from build123d import *

# Parameters (mm, degrees)
SKETCH_1_R      = 6
EXTRUDE_1_DEPTH = 3
SKETCH_2_R      = 3
EXTRUDE_2_DEPTH = 15.8
FILLET_1_R      = 1
FILLET_2_R      = 1.5


with BuildPart() as part:
    # ｽｹｯﾁ1 → ﾎﾞｽ - 押し出し1 (new body)
    with BuildSketch(Plane(origin=(0, 0, 0), x_dir=(1, 0, 0), z_dir=(0, 1, 0))):
        Circle(SKETCH_1_R)
    extrude(amount=EXTRUDE_1_DEPTH)

    # ｽｹｯﾁ2 → ﾎﾞｽ - 押し出し2 (add)
    with BuildSketch(Plane(origin=(0, 3, 0), x_dir=(1, 0, 0), z_dir=(0, 1, 0))):
        Circle(SKETCH_2_R)
    extrude(amount=EXTRUDE_2_DEPTH)

    # ﾌｨﾚｯﾄ1
    fillet_1_edges = [part.edges().sort_by_distance(p)[0] for p in [
        (-3, 18.8, 0),
    ]]
    fillet(fillet_1_edges, radius=FILLET_1_R)

    # ﾌｨﾚｯﾄ2
    fillet_2_edges = [part.edges().sort_by_distance(p)[0] for p in [
        (-6, 0, 0),
    ]]
    fillet(fillet_2_edges, radius=FILLET_2_R)


solid = part.part
For this review, take the finished solid that the model builds, in its own axes (mm). A direction names the side the tool comes from. Round coordinates to 2 decimals unless told otherwise and drop trailing zeros. Write each loop counter-clockwise with the first axis right and the second up, starting at its lowest first coordinate (ties: lowest second). Pieces come first, ordered by that corner, then holes. Notation, with made-up numbers: M 78,-22.75 L 85,-22.75 A25 cw 85,-5.75 Z; hole C 62,36 d11. An arc over 180 degrees is marked long. Write item = value, one per line. Start each with the question number.
(1) For faces 1 (the face through (-3, 3, 1)), 2 (the face through (0, 0, 0)), list the 3-axis set-ups (+Z, -Z, +X, -X, +Y, -Y) from which the entire face can be reached by the end or side of a thin tool; tool diameter is ignored.
(2) We need section A-A (x = 0). Give the boundary of the cut face in (y, z).
(3) We need section C-C (y = 15). Give the boundary of the cut face in (x, z), then the cut area to 3 significant figures.
(4) For line 1 along X through (y, z) = (6, 0); line 2 along Y through (x, z) = (3.5, -3); line 3 along Y through (x, z) = (0.75, -2.25), list the stretches that pass through material, from the lowest coordinate up.
(5) We need section B-B (z = 0). Give the boundary of the cut face in (x, y).
(6) Clearance check with flat-ended pins moving along their axes: pin 1 Ø1 at (x, z) = (1.5, -0.5) entering from -Y; pin 2 Ø4 at (x, y) = (4.5, 2.5) entering from -Z; pin 3 Ø3 at (y, z) = (3.5, -2) entering from -X; pin 4 Ø2 at (x, y) = (3, 9) entering from -Z. State where each tip first meets the part, or that it passes through.
Results found:
q1.face_1 = +Y
q1.face_2 = +Z, -Z, +X, -X, -Y
q2.outline = M 0,-4.5 A1.5 ccw 1.5,-6 L 3,-6 L 3,-3 L 17.8,-3 A1 ccw 18.8,-2 L 18.8,2 A1 ccw 17.8,3 L 3,3 L 3,6 L 1.5,6 A1.5 ccw 0,4.5 Z
q3.outline = C 0,0 d6
q3.area = 28.3 mm²
q4.line_1 = -3 to 3
q4.line_2 = 0 to 3
q4.line_3 = 0 to 18.73
q5.outline = M -6,1.5 A1.5 ccw -4.5,0 L 4.5,0 A1.5 ccw 6,1.5 L 6,3 L 3,3 L 3,17.8 A1 ccw 2,18.8 L -2,18.8 A1 ccw -3,17.8 L -3,3 L -6,3 Z
q6.pin_1 = 0
q6.pin_2 = -5.45
q6.pin_3 = -5.97
q6.pin_4 = -2.24
